The drawing under review shows one solid part. Ordinate dimensions are in mm from its lowest x, y, z. Coordinates: 2 decimals unless noted, no trailing zeros. Loops run counter-clockwise (first coordinate to the right, second up) from the corner with the lowest first, then second, coordinate; pieces in that order, holes last. Notation, with made-up numbers: (21, -16.75) -> (27, -16.75) arc R24 ccw to (27, -4.75) -> close; hole circle Ø1 at (44, 77). An arc over 180 degrees is marked (long way). Use a Markdown table: item, result.
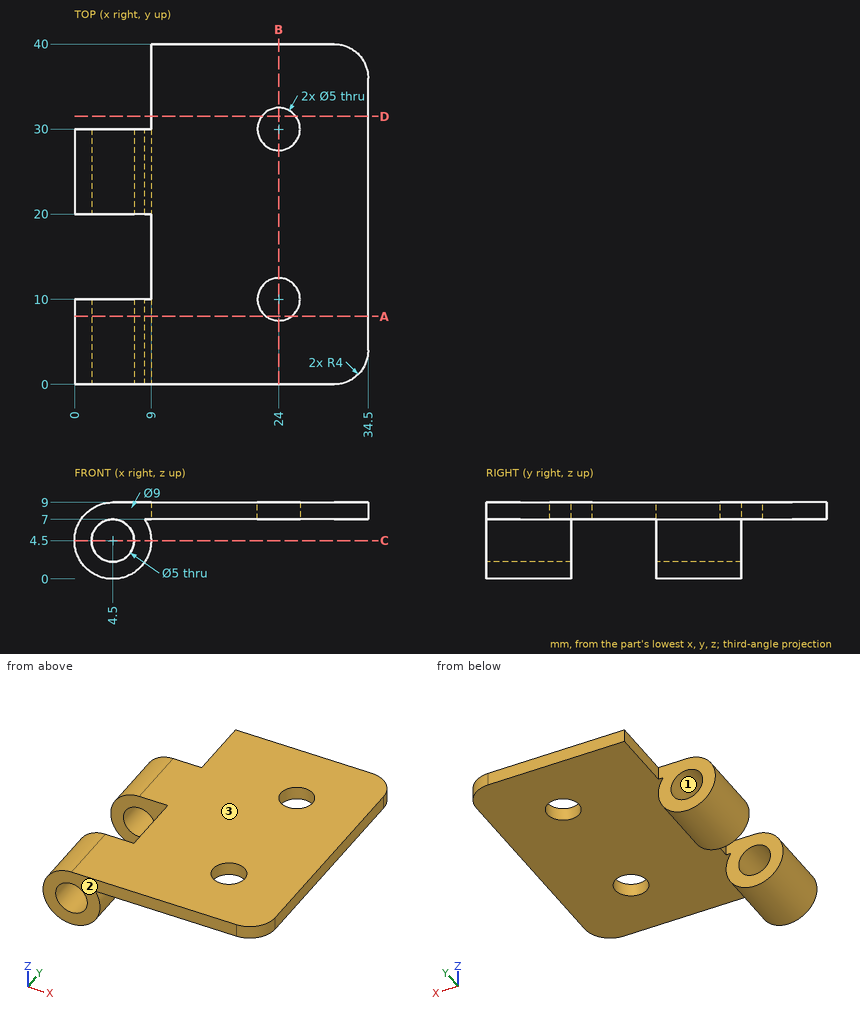
(1) Take a section at C-C on z = 4.5. Write out the cut boundary in (x, y), plus the area to 3 significant figures.
Found:
| item | result |
|---|---|
| outline | (0, 0) -> (2, 0) -> (2, 10) -> (0, 10) -> close; (0, 20) -> (2, 20) -> (2, 30) -> (0, 30) -> close; (7, 0) -> (9, 0) -> (9, 10) -> (7, 10) -> close; (7, 20) -> (9, 20) -> (9, 30) -> (7, 30) -> close |
| area | 80.0 mm^2 |
(2) Mouldability with a two-part tool opening along Z and no side actions: class the marked faces 1, 2 and 3 as pulls with the +Z half, pulls with the -Z half, needs draft (parallel to the pull), parting line crosses it, or undercut.
Found:
| item | result |
|---|---|
| face 1 | undercut |
| face 2 | needs draft |
| face 3 | pulls with the +Z half |
(3) Take a section at D-D on y = 31.5. Write out the cut boundary in (x, z), plus the area to 3 significant figures.
Found:
| item | result |
|---|---|
| outline | (9, 7) -> (22, 7) -> (22, 9) -> (9, 9) -> close; (26, 7) -> (34.5, 7) -> (34.5, 9) -> (26, 9) -> close |
| area | 43.0 mm^2 |
(4) Take a section at A-A on y = 8. Write out the cut boundary in (x, z).
Found:
| item | result |
|---|---|
| outline | (4.5, 9) arc R4.5 ccw (long way) to (8.24, 7) -> (22.5, 7) -> (22.5, 9) -> close; (25.5, 7) -> (34.5, 7) -> (34.5, 9) -> (25.5, 9) -> close; hole circle Ø5 at (4.5, 4.5) |
(5) Take a section at B-B on x = 24. Write out the cut boundary in (y, z).
Found:
| item | result |
|---|---|
| outline | (0, 7) -> (7.5, 7) -> (7.5, 9) -> (0, 9) -> close; (12.5, 7) -> (27.5, 7) -> (27.5, 9) -> (12.5, 9) -> close; (32.5, 7) -> (40, 7) -> (40, 9) -> (32.5, 9) -> close |
(6) For line 1 along Y through (x, z) = (24, 8.1); line 2 along X through (y, z) = (7.75, 4.5); line 3 along Y through (x, z) = (1.5, 4.75), list the stretches that pass through material, from the lowest coordinate up.
Found:
| item | result |
|---|---|
| line 1 | y = 0 to 7.5, 12.5 to 27.5, 32.5 to 40 |
| line 2 | x = 0 to 2, 7 to 9 |
| line 3 | y = 0 to 10, 20 to 30 |
(7) For pin 1 Ø13 at (x, y) = (16, 23.5) entering from -Z; pin 2 Ø5 at (y, z) = (29, 4) entering from +X; pin 3 Ø2.5 at (x, z) = (4, 6.5) entering from +Y, all flat-tipped, find the tip position at first contact; note any pin that passes through.
Found:
| item | result |
|---|---|
| pin 1 | stops at z = 7 |
| pin 2 | stops at x = 9 |
| pin 3 | stops at y = 30 |
